The listing builds one solid part. Answer for the finished solid, in the listing's coordinates (mm). A direction names the side the tool comes from. Round coordinates to 2 decimals unless told otherwise and drop trailing zeros. Loops run counter-clockwise (first coordinate to the right, second up) from the corner with the lowest first, then second, coordinate; pieces in that order, holes last. Notation, with made-up numbers: (-24, -25) -> (-13, -25) arc R31 cw to (-13, 12) -> close; hole circle Ø9 at (0, 32). An arc over 180 degrees is marked (long way). Write each question's results on one line, items separated by ' | '. Start each with the question number.
from build123d import *

# Parameters (mm, degrees)
F1_DEPTH = 8
F2_R     = 1.1
F3_DEPTH = 1
F4_R     = 0.75
F5_DEPTH = 2


with BuildPart() as f1:
    # F0 (on Front) → F1 (new body)
    with BuildSketch(Plane.XZ):
        with BuildLine():
            ThreePointArc((2.5, 0), (0, 2.5), (-2.5, 0))
            Line((-2.5, 0), (-2.5, -2.5))
            Line((-2.5, -2.5), (2.5, -2.5))
            Line((2.5, -2.5), (2.5, 0))
        make_face()
    extrude(amount=F1_DEPTH)

    # F2 (on face) → F3 (join)
    with BuildSketch(Plane.XZ.offset(8)):
        Circle(F2_R)
    extrude(amount=F3_DEPTH)

    # F4 (on face) → F5 (join)
    with BuildSketch(Plane.XZ.offset(9)):
        Circle(F4_R)
    extrude(amount=F5_DEPTH)


solid = f1.part
Item 1: The part is cut by section D-D, the plane x = -2.05. Give the vertices of the cut face in (y, z).
Item 2: The part is cut by section B-B, the plane y = -5. Give the vertices of the cut face in (x, z), plus the area to 3 significant figures.
Item 3: The part is cut by section C-C, the plane x = -0.95. Give the vertices of the cut face in (y, z).
Item 4: For faces 1 (the cylindrical face through (0.1, -3.9, 2.5)), 2 (the cylindrical face through (1.05, -8.49, 0.33)), determine the directions among +Z, -Z, +X, -X, +Y, -Y from which every point of the face is accessible in a straight line to the end or side of a thin tool.
Item 5: Each of these flat-tipped pins is pushed along its axis until it touches: pin 1 Ø2 at (y, z) = (-8.5, 2) entering from +X; pin 2 Ø2 at (x, y) = (-2, -5.5) entering from +Z. Where does it stop, or does it pass through?
Item 6: The part is cut by section A-A, the plane x = 0. Give the vertices of the cut face in (y, z), plus the area to 3 significant figures.
Item 7: Straight lines are drawn through the part: L1, parallel to Y at x = -1.4, z = -1.65; L2, parallel to Y at x = -0.6, z = -0.7; L3, parallel to Z at x = 0.25, y = -1.5. For each, find the intervals that lie inside material, in ascending order. Write a range as [from, to].
Report:
1) outline: (-8, -2.5) -> (0, -2.5) -> (0, 1.43) -> (-8, 1.43) -> close
2) outline: (-2.5, -2.5) -> (2.5, -2.5) -> (2.5, 0) arc R2.5 ccw to (-2.5, 0) -> close | area: 22.3 mm2
3) outline: (-9, -0.55) -> (-8, -0.55) -> (-8, -2.5) -> (0, -2.5) -> (0, 2.31) -> (-8, 2.31) -> (-8, 0.55) -> (-9, 0.55) -> close
4) face 1: +Z, +Y, -Y | face 2: -Y
5) pin 1: stops at x = 2.23 | pin 2: stops at z = 2.29
6) outline: (-11, -0.75) -> (-9, -0.75) -> (-9, -1.1) -> (-8, -1.1) -> (-8, -2.5) -> (0, -2.5) -> (0, 2.5) -> (-8, 2.5) -> (-8, 1.1) -> (-9, 1.1) -> (-9, 0.75) -> (-11, 0.75) -> close | area: 45.2 mm2
7) L1: y = [-8, 0] | L2: y = [-9, 0] | L3: z = [-2.5, 2.49]
